CAD build for the part. Positions are in the model's coordinates, mm. A direction names the side the tool comes from. Give positions to 0.01 mm unless a question says otherwise; leave off trailing zeros. Loops run counter-clockwise (first coordinate to the right, second up) from the corner with the lowest first, then second, coordinate; pieces in that order, holes last.
Item 1: Which spindle directions (+Z, -Z, +X, -X, +Y, -Y) get a long thin tool onto all of the face, cutting with end or side? Do faces 4 (the flat face through (26, 6.7, 0.4)), 5 (the flat face through (0, 1, -6)), 6 (the cylindrical face through (0.07, 2.03, -15.5)). Say none if no direction does.
Item 2: Saw through at C-C on x = 0. Give the cut face in (y, z), plus the area to 3 significant figures.
Item 3: Probe probe 1 along X at (y, z) = (1.75, 0); probe 2 along X at (y, z) = (6.5, 16); probe 3 along Y at (x, z) = (27.95, -16). List the from-to ranges inside material, lowest first.
Item 4: Saw through at B-B on z = 0. Give the cut face in (x, y).
Item 5: Saw through at A-A on y = 5.5. Give the cut face in (x, z), plus the area to 3 significant figures.
Item 6: Mould opens along Z. For faces 1 (the flat face through (28, 14, 0)), 2 (the cylindrical face through (-10, 0.5, -9.8)), 3 (the flat face through (0, 2, 25)) say: released by +Z, released by -Z, zero draft, split by the parting line, or undercut.
Item 7: Drop flat-ended pins along their axis: P1, Ø10, axis at x = -14.5, z = 5.5, coming from the -Y side; P2, Ø1.8, axis at x = -14, z = 0, coming from the -Y side; P3, Ø5, axis at x = 16.5, z = 8, coming from the +Y side; P4, Ø8.5, axis at x = 3.5, z = 0, coming from the -Y side. Give the stop position or say it passes through.
Item 8: Saw through at D-D on y = 9. Give the number of separate pieces and of enclosed holes in the cut face, plus the area to 3 significant figures.
from build123d import *

# Parameters (mm, degrees)
EXTRUDE_1_DEPTH     = 25
SKETCH_3_R          = 5
SKETCH_3_R_2        = 1.5
CUT_EXTRUDE_2_DEPTH = 4
SKETCH_4_R          = 14
CUT_EXTRUDE_3_DEPTH = 1
SKETCH_2_R          = 2
CUT_EXTRUDE_4_DEPTH = 67.49060084


with BuildPart() as part:
    # 草图1 → 凸台-拉伸1 (new, symmetric)
    with BuildSketch(Plane.XY):
        Polygon((30, 0), (-30, 0), (-30, 14), (-26, 14), (-26, 4), (26, 4), (26, 14), (30, 14), align=None)
    extrude(amount=EXTRUDE_1_DEPTH, both=True)

    # 草图3 → 切除-拉伸2 (cut)
    with BuildSketch(Plane(origin=(0, 4, 0), x_dir=(1, 0, 0), z_dir=(0, 1, 0))):
        with Locations(Location((0, 0, 0), (0, 0, 270))):
            Circle(SKETCH_3_R)
        with Locations(Location((0, 14, 0), (0, 0, 270))):
            Circle(SKETCH_3_R_2)
        with Locations(Location((14, 0, 0), (0, 0, 270))):
            Circle(SKETCH_3_R_2)
        with Locations(Location((0, -14, 0), (0, 0, 270))):
            Circle(SKETCH_3_R_2)
        with Locations(Location((-14, 0, 0), (0, 0, 270))):
            Circle(SKETCH_3_R_2)
    extrude(amount=-CUT_EXTRUDE_2_DEPTH, mode=Mode.SUBTRACT)

    # 草图4 → 切除-拉伸3 (cut)
    with BuildSketch(Plane.XZ):
        Circle(SKETCH_4_R)
    extrude(amount=-CUT_EXTRUDE_3_DEPTH, mode=Mode.SUBTRACT)

    # 草图2 → 切除-拉伸4 (cut, through all)
    with BuildSketch(Plane(origin=(30, 0, 0), x_dir=(0, 0, -1), z_dir=(1, 0, 0))):
        with Locations((-16, 9)):
            Circle(SKETCH_2_R)
        with Locations((0, 9)):
            Circle(SKETCH_2_R)
        with Locations((16, 9)):
            Circle(SKETCH_2_R)
    extrude(amount=-CUT_EXTRUDE_4_DEPTH, mode=Mode.SUBTRACT)


solid = part.part
Results below:
1. face 4: +Z, -Z, +Y
1. face 5: -Y
1. face 6: +Y, -Y
2. outline: (0, -25) - (4, -25) - (4, -15.5) - (0, -15.5) - close; (0, 15.5) - (4, 15.5) - (4, 25) - (0, 25) - close; (1, -12.5) - (4, -12.5) - (4, -5) - (1, -5) - close; (1, 5) - (4, 5) - (4, 12.5) - (1, 12.5) - close
2. area: 121 mm2
3. probe 1: x = -30 to -15.5, -12.5 to -5, 5 to 12.5, 15.5 to 30
3. probe 2: x = -30 to -26, 26 to 30
3. probe 3: y = 0 to 7, 11 to 14
4. outline: (-30, 0) - (-15.5, 0) - (-15.5, 4) - (-26, 4) - (-26, 7) - (-30, 7) - close; (-30, 11) - (-26, 11) - (-26, 14) - (-30, 14) - close; (-12.5, 1) - (-5, 1) - (-5, 4) - (-12.5, 4) - close; (5, 1) - (12.5, 1) - (12.5, 4) - (5, 4) - close; (15.5, 0) - (30, 0) - (30, 7) - (26, 7) - (26, 4) - (15.5, 4) - close; (26, 11) - (30, 11) - (30, 14) - (26, 14) - close
5. outline: (-30, -25) - (-26, -25) - (-26, 25) - (-30, 25) - close; (26, -25) - (30, -25) - (30, 25) - (26, 25) - close
5. area: 400 mm2
6. face 1: zero draft
6. face 2: undercut
6. face 3: released by +Z
7. P1: stops at y = 0
7. P2: passes through
7. P3: stops at y = 4
7. P4: stops at y = 1
8. separate pieces: 8
8. enclosed holes: 0
8. area: 304 mm2
